from build123d import *
from OCP.BRepAlgoAPI import BRepAlgoAPI_Cut
from OCP.TopTools import TopTools_ListOfShape

# Parameters (mm, degrees)
SKETCH1_R               = 57.15
SKETCH1_R_2             = 48.59
BOSS_EXTRUDE1_DEPTH     = 245.75
CUT_EXTRUDE1_DEPTH      = 57.875
CUT_EXTRUDE2_REACH      = 260.699
CUT_EXTRUDE2_END_RADIUS = 57.15
SKETCH3_R               = 22.25


with BuildPart() as part:
    # Sketch1 → Boss-Extrude1 (new body)
    with BuildSketch(Plane(origin=(0, 0, 0), x_dir=(1, 0, 0), z_dir=(0, 1, 0))):
        with Locations(Location((0, 0, 0), (0, 0, 270))):
            Circle(SKETCH1_R)
        with Locations(Location((0, 0, 0), (0, 0, 270))):
            Circle(SKETCH1_R_2, mode=Mode.SUBTRACT)
    extrude(amount=BOSS_EXTRUDE1_DEPTH)


with BuildPart() as cut_extrude1_tool:
    # Sketch2 → Cut-Extrude1 (new, symmetric)
    with BuildSketch(Plane.XY):
        with BuildLine():
            Line((57.15, 245.75), (-57.15, 245.75))
            ThreePointArc((-57.15, 245.75), (0, 238.645023145), (57.15, 245.75))
        make_face()
    extrude(amount=CUT_EXTRUDE1_DEPTH, both=True)


with BuildPart() as part_1:
    add(part.part)

    # Cut-Extrude1: cut by cut_extrude1_tool, with a tolerance
    cut_extrude1_stock = TopTools_ListOfShape()
    cut_extrude1_stock.Append(part_1.part.wrapped)
    cut_extrude1_tools = TopTools_ListOfShape()
    cut_extrude1_tools.Append(cut_extrude1_tool.part.wrapped)
    cut_extrude1_cut = BRepAlgoAPI_Cut()
    cut_extrude1_cut.SetArguments(cut_extrude1_stock)
    cut_extrude1_cut.SetTools(cut_extrude1_tools)
    cut_extrude1_cut.SetFuzzyValue(0.00001)
    cut_extrude1_cut.Build()
    add(Compound.cast(cut_extrude1_cut.Shape()).solids(), mode=Mode.REPLACE)

    # Cut-Extrude2: up to this cylinder (the profile starts inside it)
    cut_extrude2_end = Plane(origin=(0, 100, 0), z_dir=(0, -1, 0)) * Cylinder(CUT_EXTRUDE2_END_RADIUS, 636.698, mode=Mode.PRIVATE)
    # Sketch3 → Cut-Extrude2 (cut, up to the surface)
    with BuildSketch(Plane(origin=(0, 0, 0), x_dir=(0, 0, -1), z_dir=(1, 0, 0)), mode=Mode.PRIVATE) as cut_extrude2_sk1:
        with Locations(Location((0, 100, 0), (0, 0, 180))):
            Circle(SKETCH3_R)
    cut_extrude2_tool1 = extrude(cut_extrude2_sk1.sketch, amount=CUT_EXTRUDE2_REACH, mode=Mode.PRIVATE) & cut_extrude2_end
    add(cut_extrude2_tool1.solids().sort_by_distance((0, 100, 0))[0], mode=Mode.SUBTRACT)


solid = part_1.part
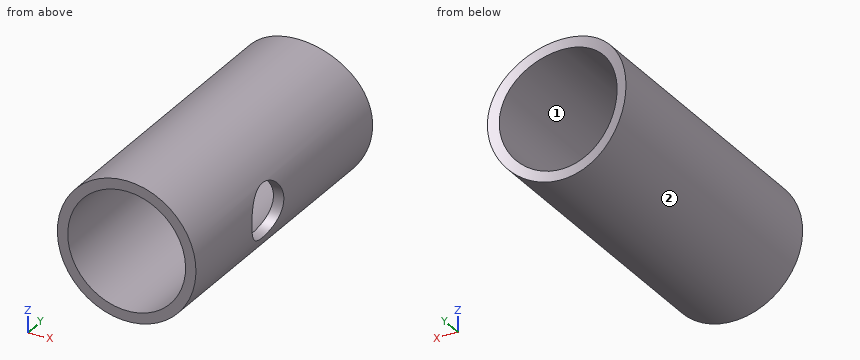
Work out the finished part from the listing and answer in its coordinate system (mm). Face numbers are marked on the shaded views. Round coordinates to 2 decimals unless told otherwise and drop trailing zeros. Loops run counter-clockwise (first coordinate to the right, second up) from the corner with the lowest first, then second, coordinate; pieces in that order, holes last. Notation, with made-up numbers: (80, 15) -> (87, 15) arc R14 ccw to (87, 19) -> close; hole circle Ø1 at (34.25, 17.25). An arc over 180 degrees is marked (long way). Use one line per item in the form item = value.
(1) Straight lines are drawn through the part: line 1 (X direction, y = 59, z = 0); line 2 (Y direction, x = -48.5, z = -5). For each, find the intervals that lie inside material, in ascending order.
Answer list:
line_1 = -57.15 to -48.59, 48.59 to 57.15
line_2 = 0 to 243.74
(2) Find section B-B on z = 0. Give the vertices of the cut face in (x, y).
Answer list:
outline = (-57.15, 0) -> (-48.59, 0) -> (-48.59, 243.76) arc R233.4 cw to (-57.15, 245.75) -> close; (48.59, 0) -> (57.15, 0) -> (57.15, 77.75) -> (48.59, 77.75) -> close; (48.59, 122.25) -> (57.15, 122.25) -> (57.15, 245.75) arc R233.4 cw to (48.59, 243.76) -> close
(3) Find section C-C on z = -31.5. Give the vertices of the cut face in (x, y).
Answer list:
outline = (-47.69, 0) -> (-37, 0) -> (-37, 241.6) arc R233.4 cw to (-47.69, 243.57) -> close; (37, 0) -> (47.69, 0) -> (47.69, 243.57) arc R233.4 cw to (37, 241.6) -> close
(4) Flat-ended cylindrical pins translate along their axes: P1, Ø1, axis at x = 42.5, z = 40.5, coming from the -Y side; P2, Ø2, axis at y = 175, z = 28.5, coming from the +X side; P3, Ø1, axis at y = 122, z = 1, coming from the -X side; P4, Ø6, axis at y = 65.5, z = -15.5, coming from the -X side. Find the tip coordinate at first contact, or state that the pin passes through.
Answer list:
P1 = through
P2 = 50.1
P3 = -57.15
P4 = -55.77
(5) For a pull along Z with two mould halves and no side action, classify the marked faces 1 and 2 as released by +Z, released by -Z, zero draft, split by the parting line, or undercut.
Answer list:
face_1 = undercut
face_2 = split by the parting line
(6) Find section A-A on x = 0. Give the vertices of the cut face in (y, z).
Answer list:
outline = (0, -57.15) -> (238.65, -57.15) -> (238.65, -48.59) -> (0, -48.59) -> close; (0, 48.59) -> (238.65, 48.59) -> (238.65, 57.15) -> (0, 57.15) -> close
(7) Find section D-D on x = 46. Give the vertices of the cut face in (y, z).
Answer list:
outline = (0, -33.91) -> (243.22, -33.91) -> (243.22, -15.65) -> (115.81, -15.65) arc R22.25 cw to (84.19, -15.65) -> (0, -15.65) -> close; (0, 15.65) -> (84.19, 15.65) arc R22.25 cw to (115.81, 15.65) -> (243.22, 15.65) -> (243.22, 33.91) -> (0, 33.91) -> close
